from build123d import *

# Parameters (mm, degrees)
SKETCH1_R           = 1.1
SKETCH1_W           = 41
SKETCH1_H           = 21
BOSS_EXTRUDE1_DEPTH = 11
SKETCH2_R           = 9.000000034
BOSS_EXTRUDE2_DEPTH = 2


with BuildPart() as part:
    # Sketch1 → Boss-Extrude1 (new body)
    with BuildSketch(Plane.XY):
        with BuildLine():
            Line((4, -5.500000004), (37, -5.500000004))
            ThreePointArc((37, -5.500000004), (53.000000004, 10.5), (37, 26.500000004))
            Line((37, 26.500000004), (4, 26.500000004))
            ThreePointArc((4, 26.500000004), (-12.000000004, 10.5), (4, -5.500000004))
        make_face()
        with Locations((-3.5, 15.5)):
            Circle(SKETCH1_R, mode=Mode.SUBTRACT)
        with Locations((-3.5, 5.5)):
            Circle(SKETCH1_R, mode=Mode.SUBTRACT)
        with Locations((44.5, 5.5)):
            Circle(SKETCH1_R, mode=Mode.SUBTRACT)
        with Locations((44.5, 15.5)):
            Circle(SKETCH1_R, mode=Mode.SUBTRACT)
        with Locations((20.5, 10.5)):
            Rectangle(SKETCH1_W, SKETCH1_H, mode=Mode.SUBTRACT)
    extrude(amount=BOSS_EXTRUDE1_DEPTH)

    # Sketch2 → Boss-Extrude2 (add)
    with BuildSketch(Plane.XY):
        with BuildLine():
            Line((37, 26.500000004), (4, 26.500000004))
            ThreePointArc((4, 26.500000004), (-12.000000004, 10.5), (4, -5.500000004))
            Line((4, -5.500000004), (37, -5.500000004))
            ThreePointArc((37, -5.500000004), (53.000000004, 10.5), (37, 26.500000004))
        make_face()
        with Locations((30.749999966, 10.5)):
            Circle(SKETCH2_R, mode=Mode.SUBTRACT)
    extrude(amount=-BOSS_EXTRUDE2_DEPTH)


solid = part.part
Verification items for the finished model (mm, model axes). A direction names the side the tool comes from. Coordinates: 2 decimals unless noted, no trailing zeros. Order: outer loops, then holes, each group sorted by start corner. A loop starts at its lowest first (then second) coordinate and runs counter-clockwise, first axis right, second up.
Item 1: Section check D-D, the plane x = 9.5. Enter the section's corners in (y, z).
Filled in:
outline: (-5.5, -2) - (26.5, -2) - (26.5, 11) - (21, 11) - (21, 0) - (0, 0) - (0, 11) - (-5.5, 11) - close
Item 2: Release check for a two-part mould opening along Y. For faces 3 (the face through (-11.996, 10.852, 4.591)), 4 (the face through (21, 26.5, 5)), 5 (the face through (-4, 16, 0)) record: +Y half, -Y half, draft (parallel to the pull), parting line (faces both ways), or undercut.
Filled in:
face 3: parting line
face 4: +Y half
face 5: undercut
Item 3: Section check B-B, the plane x = 30.75. Enter the section's corners in (y, z).
Filled in:
outline: (-5.5, -2) - (1.5, -2) - (1.5, 0) - (0, 0) - (0, 11) - (-5.5, 11) - close; (19.5, -2) - (26.5, -2) - (26.5, 11) - (21, 11) - (21, 0) - (19.5, 0) - close
Item 4: Depth check by flat-ended pin: pin 1 (16 mm diameter, centred on x = 30.75, y = 10.5, fed in from +Z); pin 2 (1.3 mm diameter, centred on x = 44.5, y = 15.5, fed in from +Z); pin 3 (3.5 mm diameter, centred on y = 15, z = 3.5, fed in from -X); pin 4 (2 mm diameter, centred on x = 45, z = 0, fed in from -Y). Enter the tip coordinate at first touch or a pass-through.
Filled in:
pin 1: passes through
pin 2: stops at z = 0
pin 3: stops at x = -11.76
pin 4: stops at y = -3.89
Item 5: Material ranges on L1, parallel to Y at x = -3.5, z = 6.5; L2, parallel to Y at x = 45, z = 3.75; L3, parallel to X at y = 11, z = 5, recorded low to high.
Filled in:
L1: y = -3.63 to 4.4, 6.6 to 14.4, 16.6 to 24.63
L2: y = -3.36 to 4.52, 6.48 to 14.52, 16.48 to 24.36
L3: x = -11.99 to 0, 41 to 52.99
Item 6: Section check A-A, the plane y = 10.5. Enter the section's corners in (x, z).
Filled in:
outline: (-12, -2) - (21.75, -2) - (21.75, 0) - (0, 0) - (0, 11) - (-12, 11) - close; (39.75, -2) - (53, -2) - (53, 11) - (41, 11) - (41, 0) - (39.75, 0) - close
Item 7: Access from +Z, -Z, +X, -X, +Y, -Y to the whole of each face (thin tool, end or side, straight path). Record for faces 1 (the face through (20, -5.5, 5)), 2 (the face through (-2.45, 5.83, 5.42)).
Filled in:
face 1: +Z, -Z, +X, -X, -Y
face 2: +Z
Item 8: Section check C-C, the plane z = 7.5. Enter the section's corners in (x, y), then the cut area to 3 significant figures.
Filled in:
outline: (4, -5.5) - (37, -5.5) arc R16 ccw to (37, 26.5) - (4, 26.5) arc R16 ccw to start; hole circle Ø2.2 at (-3.5, 5.5); hole circle Ø2.2 at (-3.5, 15.5); hole (0, 0) - (41, 0) - (41, 21) - (0, 21) - close; hole circle Ø2.2 at (44.5, 5.5); hole circle Ø2.2 at (44.5, 15.5)
area: 984 mm2
